Input: dimensioned drawing with shaded views. Units: mm. Origin: part minimum x, y, z. A direction names the side the tool comes from. Round coordinates to 2 decimals unless told otherwise and drop trailing zeros. Loops run counter-clockwise (first coordinate to the right, second up) from the corner with the lowest first, then second, coordinate; pieces in that order, holes last. Notation, with made-up numbers: M -18.75,30.5 L 2.25,30.5 A19 ccw 2.25,65.5 Z; hole C 80,-1 d4. An arc over 180 degrees is marked long. Answer as a JSON object with one key per item and string values.
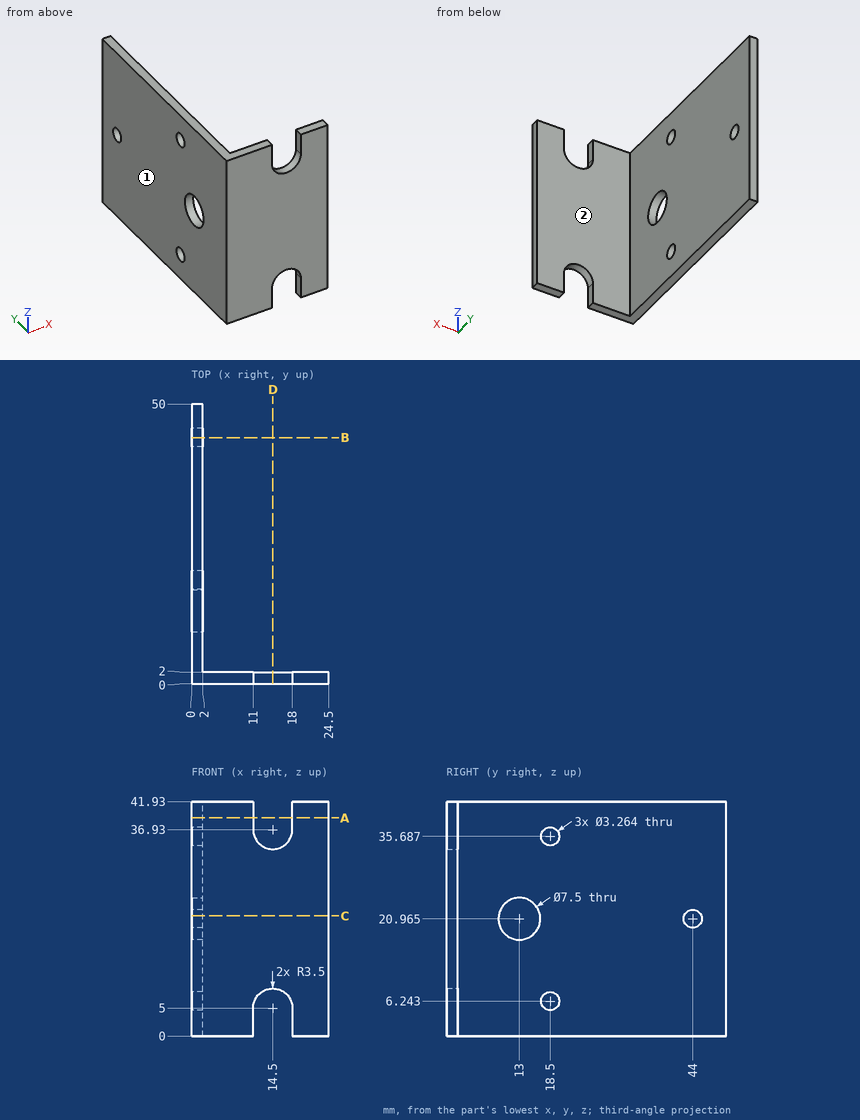
Item 1: Section B-B on y = 44. Return the cut outline in (x, z).
Answer sheet:
{"outline": "M 0,0 L 2,0 L 2,19.33 L 0,19.33 Z; M 0,22.6 L 2,22.6 L 2,41.93 L 0,41.93 Z"}
Item 2: Section A-A on z = 39. Return the cut outline in (x, y), then the cut area to 3 significant figures.
Answer sheet:
{"outline": "M 0,0 L 11,0 L 11,2 L 2,2 L 2,50 L 0,50 Z; M 18,0 L 24.5,0 L 24.5,2 L 18,2 Z", "area": "131 mm²"}
Item 3: Section C-C on z = 21.5. Return the cut outline in (x, y).
Answer sheet:
{"outline": "M 0,0 L 24.5,0 L 24.5,2 L 2,2 L 2,9.29 L 0,9.29 Z; M 0,16.71 L 2,16.71 L 2,42.46 L 0,42.46 Z; M 0,45.54 L 2,45.54 L 2,50 L 0,50 Z"}
Item 4: Line query: probe 1 along X at (y, z) = (44.5, 25). Output: solid intervals per line, ascending. Write a range as from..to.
Answer sheet:
{"probe 1": "x = 0..2"}
Item 5: Contact query for flat-ended pins moving along their axis: pin 1 Ø10 at (y, z) = (23, 10) entering from +X; pin 2 Ø1 at (x, z) = (7, 6) entering from +Y; pin 3 Ø2.5 at (y, z) = (18.5, 6.24) entering from -X. Output: stop coordinate, or through.
Answer sheet:
{"pin 1": "stops at x = 2", "pin 2": "stops at y = 2", "pin 3": "passes through"}
Item 6: Access query for the marked faces 1 and 2. Directions: +Z, -Z, +X, -X, +Y, -Y. A direction counts if a zero-diameter tool reaches every point of the face in a straight line with its end or side. Return the directions, or none.
Answer sheet:
{"face 1": "+Z, -Z, -X, +Y, -Y", "face 2": "+Z, -Z, +X, +Y"}
Item 7: Section D-D on x = 14.5. Return the cut outline in (y, z).
Answer sheet:
{"outline": "M 0,8.5 L 2,8.5 L 2,33.43 L 0,33.43 Z"}
